Autodesk Inventor part; units mm, degrees
ref_plane "YZ Plane" through (0, 0, 0) normal (1, 0, 0) x (0, 1, 0)
ref_plane "XZ Plane" through (0, 0, 0) normal (0, 1, 0) x (-1, 0, 0)
ref_plane "XY Plane" through (0, 0, 0) normal (0, 0, 1) x (1, 0, 0)
sketch "Sketch1" plane through (0, 0, 0) normal (0, 0, 1) x (1, 0, 0)
  line L0 (0, 180) -> (40, 180)
  line L1 (40, 180) -> (40, 40)
  line L2 (40, 40) -> (20, 0)
  line L3 (20, 0) -> (0, 0)
  line L4 (0, 0) -> (0, 180)
  point P0 (10, 0)
  dimension "d1" = 40
  dimension "d2" = 20
  dimension "d4" = 180
  dimension "d5" = 140
revolve "Revolution1" add sketch "Sketch1" angle 360 about axis through (0, 0, 0) along (0, 1, 0)
sketch "Sketch2" plane through (0, 180, 0) normal (0, 1, 0) x (1, 0, 0)
  circle A0 centre (0, 0) radius 37
  circle A1 centre (0, 0) radius 40
  dimension "d14" = 3
extrude "Extrusion1" cut sketch "Sketch2" against normal blind 145 contours A0
sketch "Sketch3" plane through (0, 0, 0) normal (0, -1, 0) x (1, 0, 0)
  circle A0 centre (0, 0) radius 16
  circle A1 centre (0, 0) radius 20
extrude "Extrusion2" cut sketch "Sketch3" against normal blind 140 contours A0
sketch "Sketch4" plane through (0, 35, 0) normal (0, 1, 0) x (1, 0, 0)
  circle A0 centre (0, 0) radius 25
  dimension "d11" = 50
extrude "Extrusion3" cut sketch "Sketch4" against normal blind 20
sketch "Sketch5" plane through (0, 0, 0) normal (0, -1, 0) x (1, 0, 0)
  point P0 (0, 0)
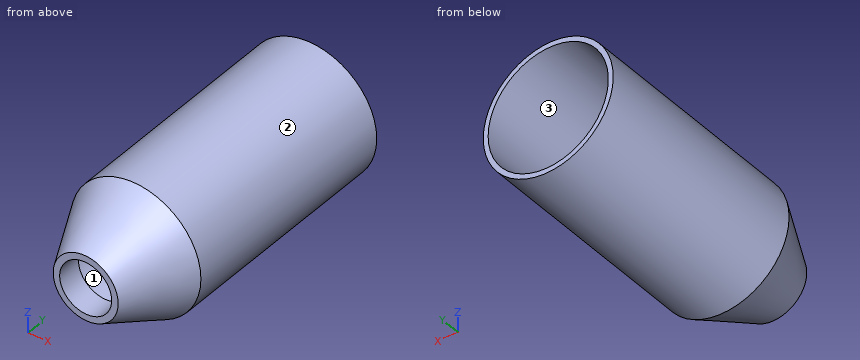
Input: part model. Units: mm. Frame: model coordinates. Face numbers are marked on the shaded views. Give positions to 0.01 mm unless a question says otherwise; leave off trailing zeros. Write each loop counter-clockwise with the first axis right and the second up, starting at its lowest first coordinate (ties: lowest second). Pieces come first, ordered by that corner, then holes. Notation, with made-up numbers: (66, -24) - (77, -24) arc R20 cw to (77, -2) - close; hole circle Ø3 at (-23.5, -17). An arc over 180 degrees is marked (long way). Write item = value, one per line. Start each with the question number.
1) Cut plane A-A (z = 0). Return loops of the section in (x, y).
2) Material intervals for L1, parallel to Z at x = 0, y = 150; L2, parallel to X at y = 134.5, z = -3.5; L3, parallel to Z at x = -34, y = 55.5, sorted ascending. Write a range as [from, to].
3) Pin query (flat end, axial travel): pin 1 (2 mm diameter, centred on y = 30, z = -9.5, fed in from +X); pin 2 (12 mm diameter, centred on x = 32, y = 35, fed in from -Z); pin 3 (5 mm diameter, centred on x = -25.5, y = 110, fed in from -Z). Return the tip coordinate at first contact, or that it passes through.
4) Cut plane C-C (y = 17). Return loops of the section in (x, z), and give its area (3 significant figures).
5) Draft query along X for the marked faces 1, 2 and 3. Return one class per face: pulls with the +X half, pulls with the -X half, needs draft (parallel to the pull), parting line crosses it, or undercut.
6) Cut plane B-B (x = 0). Return loops of the section in (y, z).
Answers follow:
q1.outline = (-40, 40) - (-20, 0) - (-16, 0) - (-16, 15) - (-25, 15) - (-25, 35) - (-37, 35) - (-37, 180) - (-40, 180) - close; (16, 0) - (20, 0) - (40, 40) - (40, 180) - (37, 180) - (37, 35) - (25, 35) - (25, 15) - (16, 15) - close
q2.L1 = [-40, -37], [37, 40]
q2.L2 = [-39.85, -36.83], [36.83, 39.85]
q2.L3 = [-21.07, -14.59], [14.59, 21.07]
q3.pin_1 = 34.27
q3.pin_2 = -28.37
q3.pin_3 = -32.73
q4.outline = circle Ø57 at (0, 0); hole circle Ø50 at (0, 0)
q4.area = 588 mm^2
q5.face_1 = undercut
q5.face_2 = parting line crosses it
q5.face_3 = undercut
q6.outline = (0, -20) - (40, -40) - (180, -40) - (180, -37) - (35, -37) - (35, -25) - (15, -25) - (15, -16) - (0, -16) - close; (0, 16) - (15, 16) - (15, 25) - (35, 25) - (35, 37) - (180, 37) - (180, 40) - (40, 40) - (0, 20) - close
